```python
from build123d import *

# Parameters (mm, degrees)
F0_R     = 2
F1_DEPTH = 25
F2_R     = 4
F2_R_2   = 2
F3_DEPTH = 3
F4_SIZE  = 0.4


with BuildPart() as f1:
    # F0 (on Top) → F1 (new body)
    with BuildSketch(Plane.XY):
        Circle(F0_R)
    extrude(amount=F1_DEPTH)

    # F2 (on face) → F3 (join)
    with BuildSketch(Plane.XY.offset(25)):
        Circle(F2_R)
        Circle(F2_R_2, mode=Mode.SUBTRACT)
        Circle(F2_R_2)
    extrude(amount=F3_DEPTH)

    # F4
    f4_edges = [f1.edges().sort_by_distance(p)[0] for p in [
        (-4, 0, 28),
        (-4, 0, 25),
    ]]
    chamfer(f4_edges, length=F4_SIZE)


solid = f1.part
```
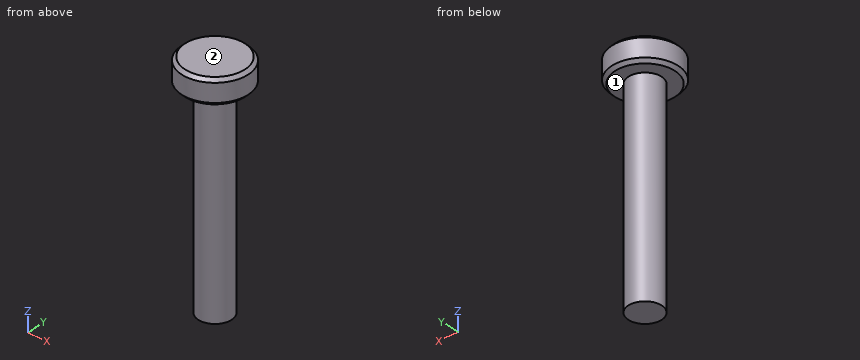
The listing builds one solid part. Answer for the finished solid, in the listing's coordinates (mm). Face numbers are marked on the shaded views. A direction names the side the tool comes from. Coordinates: 2 decimals unless noted, no trailing zeros. Loops run counter-clockwise (first coordinate to the right, second up) from the corner with the lowest first, then second, coordinate; pieces in that order, holes last. Notation, with made-up numbers: (63.25, 24.25) -> (88.25, 24.25) arc R32 ccw to (88.25, 50.25) -> close; hole circle Ø8 at (14, 26). An arc over 180 degrees is marked (long way). Return JSON: item names as keys, results as strings. Group by question number.
(1) A cutting plane is placed at A-A on x = 0. Write down the section's boundary in (y, z), and give its area (3 significant figures).
(2) A cutting plane is placed at C-C on z = 17.75. Write down the section's boundary in (x, y).
(3) Find the intervals of material crossed by probe 1 along Z at (x, y) = (1.75, 1.5); probe 2 along X at (y, z) = (0.75, 3.5); probe 3 along Y at (x, z) = (0, 12.25), in increasing order. Write a range as from..to.
(4) Given pin 1 Ø1.5 at (x, z) = (-2, 8) entering from +Y; pin 2 Ø3 at (y, z) = (-2, 10.5) entering from -X, each flat-ended and moving along its own axis, determine where each tip first touches the part or whether it passes through.
(5) Which of the six approach directions +Z, -Z, +X, -X, +Y, -Y give full straight-line access (tool end or side, diameter ignored) to the marked faces 1 and 2?
The answers:
{
 "1": {"outline": "(-4, 25.4) -> (-3.6, 25) -> (-2, 25) -> (-2, 0) -> (2, 0) -> (2, 25) -> (3.6, 25) -> (4, 25.4) -> (4, 27.6) -> (3.6, 28) -> (-3.6, 28) -> (-4, 27.6) -> close", "area": "124 mm^2"},
 "2": {"outline": "circle Ø4 at (0, 0)"},
 "3": {"probe 1": "z = 25..28", "probe 2": "x = -1.85..1.85", "probe 3": "y = -2..2"},
 "4": {"pin 1": "stops at y = 1.56", "pin 2": "stops at x = -1.94"},
 "5": {"face 1": "-Z", "face 2": "+Z, +X, -X, +Y, -Y"}
}
